Part model, mm, in its own coordinate system. Face numbers are marked on the shaded views. A direction names the side the tool comes from. Coordinates: 2 decimals unless noted, no trailing zeros. Order: outer loops, then holes, each group sorted by start corner. A loop starts at its lowest first (then second) coordinate and runs counter-clockwise, first axis right, second up.
```python
from build123d import *

# Parameters (mm, degrees)
BOSS_EXTRUDE1_DEPTH = 9.525
FILLET1_R           = 3.175
SKETCH2_R           = 3.302
CUT_EXTRUDE1_DEPTH  = 70.215728207
SKETCH3_R           = 3.302
CUT_EXTRUDE2_DEPTH  = 70.215728207


with BuildPart() as part:
    # Sketch1 → Boss-Extrude1 (new body)
    with BuildSketch(Plane.XY):
        Polygon((-50.8, 0), (0, 0), (0, -50.8), (-4.7625, -50.8), (-4.7625, -4.7625), (-50.8, -4.7625), align=None)
    extrude(amount=BOSS_EXTRUDE1_DEPTH)

    # Fillet1
    fillet1_edges = [part.edges().sort_by_distance(p)[0] for p in [
        (-4.7625, -50.8, 4.7625),
        (-4.7625, -4.7625, 4.7625),
        (-50.8, -4.7625, 4.7625),
    ]]
    fillet(fillet1_edges, radius=FILLET1_R)

    # Sketch2 → Cut-Extrude1 (cut, through all)
    with BuildSketch(Plane.ZY.offset(4.7625)):
        with Locations(Location((4.7625, -41.275, 0), (0, 0, 270))):
            Circle(SKETCH2_R)
        with Locations(Location((4.7625, -22.225, 0), (0, 0, 270))):
            Circle(SKETCH2_R)
    extrude(amount=-CUT_EXTRUDE1_DEPTH, mode=Mode.SUBTRACT)

    # Sketch3 → Cut-Extrude2 (cut, through all)
    with BuildSketch(Plane.XZ.offset(4.7625)):
        with Locations((-41.275, 4.7625)):
            Circle(SKETCH3_R)
        with Locations((-22.225, 4.7625)):
            Circle(SKETCH3_R)
    extrude(amount=-CUT_EXTRUDE2_DEPTH, mode=Mode.SUBTRACT)


solid = part.part
```
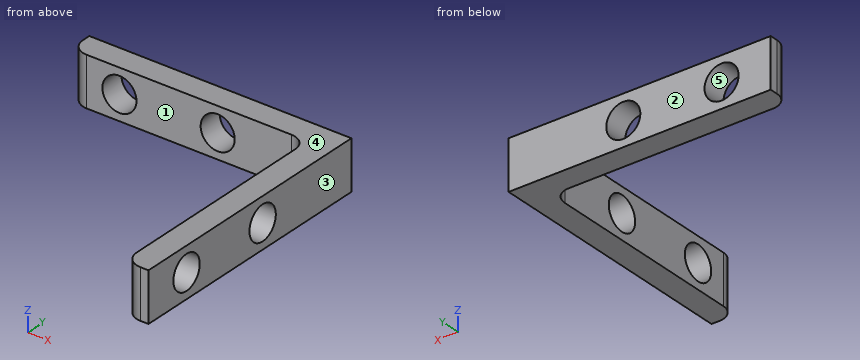
(1) Slice it at C-C, the plane x = -20.5. Give the cut face in (y, z) (1 decimal), then the cut area to 3 significant figures.
(2) Slice it at A-A, the plane z = 7.25. State how many separate pieces and enclosed holes the cut face has, then the cut area to 3 significant figures.
(3) Probe line 1 (X direction, y = -2.5, z = 3.5); line 2 (Y direction, x = -2.5, z = 5.5); line 3 (Y direction, x = -35, z = 2). List the from-to ranges inside material, lowest first.
(4) Slice it at D-D, the plane y = -47. Give the cut face in (x, z) (1 decimal).
(5) Pull direction Z, two halves, no side cores. Call the marked faces 3, 4 and 5: +Z half, -Z half, draft (parallel to the pull), parting line (faces both ways), or undercut.
(6) Drop a flat-ended pin along its axis: pin 1 (4 mm diameter, centred on y = -18.5, z = 3, fed in from -X). Give the stop position or say it passes through.
(7) Tool access for the marked faces 1 and 2: list every direction of +Z, -Z, +X, -X, +Y, -Y with a clear straight run to the whole face (end or side of a thin tool).
(8) Slice it at B-B, the plane y = -39. Give the cut face in (x, z) (1 decimal).
Here are the results:
1. outline: (-4.8, 0) - (0, 0) - (0, 1.9) - (-4.8, 1.9) - close; (-4.8, 7.6) - (0, 7.6) - (0, 9.5) - (-4.8, 9.5) - close
1. area: 18.5 mm2
2. separate pieces: 5
2. enclosed holes: 0
2. area: 376 mm2
3. line 1: x = -50.67 to -44.33, -38.22 to -25.28, -19.17 to 0
3. line 2: y = -50.67 to -44.49, -38.06 to -25.44, -19.01 to 0
3. line 3: y = -4.76 to 0
4. outline: (-4.8, 0) - (0, 0) - (0, 9.5) - (-4.8, 9.5) - close
5. face 3: draft
5. face 4: +Z half
5. face 5: undercut
6. pin 1: stops at x = -4.76
7. face 1: +Z, -Z, -X, -Y
7. face 2: +Z, -Z, +X, -X, +Y
8. outline: (-4.8, 0) - (0, 0) - (0, 2.4) - (-4.8, 2.4) - close; (-4.8, 7.2) - (0, 7.2) - (0, 9.5) - (-4.8, 9.5) - close
